Read the model definition and answer for the solid it produces. Units are mm, in the model's axes. A direction names the side the tool comes from. Coordinates: 2 decimals unless noted, no trailing zeros. Loops run counter-clockwise (first coordinate to the right, second up) from the corner with the lowest first, then second, coordinate; pieces in that order, holes last.
from build123d import *

# Parameters (mm, degrees)
SKETCH1_R           = 1.3
BOSS_EXTRUDE1_DEPTH = 2.8
BOSS_EXTRUDE2_START = -1.8
SKETCH2_R           = 1.3
BOSS_EXTRUDE2_DEPTH = 1.8
SKETCH3_R           = 2.25
CUT_EXTRUDE1_DEPTH  = 2.5
SKETCH4_W           = 35.6
SKETCH4_H           = 4.6
BOSS_EXTRUDE3_DEPTH = 5
SKETCH5_W           = 4.5
SKETCH5_H           = 35.6
BOSS_EXTRUDE4_DEPTH = 15
FILLET1_R           = 1
CUT_EXTRUDE4_DEPTH  = 3.5
SKETCH10_R          = 30
BOSS_EXTRUDE6_DEPTH = 4.5
SKETCH6_R           = 1.6
CUT_EXTRUDE2_DEPTH  = 69.491291157
SKETCH8_R           = 2.8
CUT_EXTRUDE3_DEPTH  = 2.7
RIB1_REACH          = 73.132
SKETCH11_WALL_W     = 161.35156572
SKETCH11_WALL_H     = 8
FILLET2_R           = 0.5
FILLET3_R           = 0.5


with BuildPart() as part:
    # Sketch1 → Boss-Extrude1 (new body)
    with BuildSketch(Plane(origin=(0, 0, 0), x_dir=(1, 0, 0), z_dir=(0, 1, 0))):
        Polygon((4.489988864, 12.2), (4.489988864, 17.8), (38.3, 17.8), (38.3, -17.8), (4.489988864, -17.8), (4.489988864, -12.2), (33.2, -12.2), (33.2, 12.2), align=None)
        with Locations(Location((12.5, 15, 0), (0, 0, 270))):
            Circle(SKETCH1_R, mode=Mode.SUBTRACT)
        with Locations(Location((29.5, 15, 0), (0, 0, 270))):
            Circle(SKETCH1_R, mode=Mode.SUBTRACT)
        with Locations(Location((12.5, -15, 0), (0, 0, 270))):
            Circle(SKETCH1_R, mode=Mode.SUBTRACT)
        with Locations(Location((29.5, -15, 0), (0, 0, 270))):
            Circle(SKETCH1_R, mode=Mode.SUBTRACT)
        with Locations(Location((35.75, -8.5, 0), (0, 0, 270))):
            Circle(SKETCH1_R, mode=Mode.SUBTRACT)
        with Locations(Location((35.75, 8.5, 0), (0, 0, 270))):
            Circle(SKETCH1_R, mode=Mode.SUBTRACT)
    boss_extrude1 = extrude(amount=BOSS_EXTRUDE1_DEPTH)

    # Sketch2 → Boss-Extrude2 (add)
    # profile 1 of 2: a face of its own
    with BuildSketch(Plane(origin=(0, 0, 0), x_dir=(1, 0, 0), z_dir=(0, 1, 0)).offset(BOSS_EXTRUDE2_START)):
        with BuildLine():
            ThreePointArc((4.489988864, -12.2), (13, 0), (4.489988864, 12.2))
            Line((4.489988864, 12.2), (33.2, 12.2))
            Line((33.2, 12.2), (33.2, -12.2))
            Line((33.2, -12.2), (4.489988864, -12.2))
        make_face()
    # profile 2 of 2: a face of its own
    with BuildSketch(Plane(origin=(0, 0, 0), x_dir=(1, 0, 0), z_dir=(0, 1, 0)).offset(BOSS_EXTRUDE2_START)):
        Polygon((4.489988864, 12.2), (4.489988864, 17.8), (38.3, 17.8), (38.3, -17.8), (4.489988864, -17.8), (4.489988864, -12.2), (33.2, -12.2), (33.2, 12.2), align=None)
        with Locations(Location((12.5, -15, 0), (0, 0, 270))):
            Circle(SKETCH2_R, mode=Mode.SUBTRACT)
        with Locations(Location((29.5, -15, 0), (0, 0, 270))):
            Circle(SKETCH2_R, mode=Mode.SUBTRACT)
        with Locations(Location((35.75, -8.5, 0), (0, 0, 270))):
            Circle(SKETCH2_R, mode=Mode.SUBTRACT)
        with Locations(Location((35.75, 8.5, 0), (0, 0, 270))):
            Circle(SKETCH2_R, mode=Mode.SUBTRACT)
        with Locations(Location((29.5, 15, 0), (0, 0, 270))):
            Circle(SKETCH2_R, mode=Mode.SUBTRACT)
        with Locations(Location((12.5, 15, 0), (0, 0, 270))):
            Circle(SKETCH2_R, mode=Mode.SUBTRACT)
    boss_extrude2 = extrude(amount=BOSS_EXTRUDE2_DEPTH)

    # Sketch3 → Cut-Extrude1 (cut)
    with BuildSketch(Plane.XZ.offset(1.8)):
        with Locations(Location((12.5, 15, 0), (0, 0, 270))):
            Circle(SKETCH3_R)
        with Locations(Location((29.5, 15, 0), (0, 0, 270))):
            Circle(SKETCH3_R)
        with Locations(Location((29.5, -15, 0), (0, 0, 270))):
            Circle(SKETCH3_R)
        with Locations(Location((12.5, -15, 0), (0, 0, 270))):
            Circle(SKETCH3_R)
        with Locations(Location((35.75, 8.5, 0), (0, 0, 270))):
            Circle(SKETCH3_R)
        with Locations(Location((35.75, -8.5, 0), (0, 0, 270))):
            Circle(SKETCH3_R)
    cut_extrude1 = extrude(amount=-CUT_EXTRUDE1_DEPTH, mode=Mode.SUBTRACT)

    # Sketch4 → Boss-Extrude3 (add)
    with BuildSketch(Plane(origin=(38.3, 0, 0), x_dir=(0, 0, -1), z_dir=(1, 0, 0))):
        with Locations((0, 0.5)):
            Rectangle(SKETCH4_W, SKETCH4_H)
    boss_extrude3 = extrude(amount=BOSS_EXTRUDE3_DEPTH)

    # Sketch5 → Boss-Extrude4 (add)
    with BuildSketch(Plane(origin=(0, 2.8, 0), x_dir=(1, 0, 0), z_dir=(0, 1, 0))):
        with Locations((41.05, 0)):
            Rectangle(SKETCH5_W, SKETCH5_H)
    boss_extrude4 = extrude(amount=BOSS_EXTRUDE4_DEPTH)

    # Mirror3: Boss-Extrude1, Boss-Extrude2, Cut-Extrude1, Boss-Extrude3, Boss-Extrude4 across plane
    add(boss_extrude1.mirror(Plane.ZX.offset(17.8)))
    add(boss_extrude2.mirror(Plane.ZX.offset(17.8)))
    add(cut_extrude1.mirror(Plane.ZX.offset(17.8)), mode=Mode.SUBTRACT)
    add(boss_extrude3.mirror(Plane.ZX.offset(17.8)))
    add(boss_extrude4.mirror(Plane.ZX.offset(17.8)))

    # Fillet1
    fillet1_edges = [part.edges().sort_by_distance(p)[0] for p in [
        (4.489988864, 35.1, -17.8),
        (4.489988864, 35.1, 17.8),
        (4.489988864, 0.5, 17.8),
        (4.489988864, 0.5, -17.8),
    ]]
    fillet(fillet1_edges, radius=FILLET1_R)

    # Sketch9 → Cut-Extrude4 (cut)
    with BuildSketch(Plane(origin=(43.3, 0, 0), x_dir=(0, 0, -1), z_dir=(1, 0, 0))):
        with BuildLine():
            Line((-2.05, 21.85), (2.05, 21.85))
            ThreePointArc((2.05, 21.85), (3.464213562, 21.264213562), (4.05, 19.85))
            Line((4.05, 19.85), (4.05, 15.75))
            ThreePointArc((4.05, 15.75), (3.464213562, 14.335786438), (2.05, 13.75))
            Line((2.05, 13.75), (-2.05, 13.75))
            ThreePointArc((-2.05, 13.75), (-3.464213562, 14.335786438), (-4.05, 15.75))
            Line((-4.05, 15.75), (-4.05, 19.85))
            ThreePointArc((-4.05, 19.85), (-3.464213562, 21.264213562), (-2.05, 21.85))
        make_face()
    extrude(amount=-CUT_EXTRUDE4_DEPTH, mode=Mode.SUBTRACT)

    # Sketch10 → Boss-Extrude6 (add)
    with BuildSketch(Plane.ZY.offset(-38.8)):
        with Locations((0, 17.8)):
            Circle(SKETCH10_R)
    extrude(amount=-BOSS_EXTRUDE6_DEPTH)

    # Sketch6 → Cut-Extrude2 (cut, through all)
    with BuildSketch(Plane(origin=(43.3, 0, 0), x_dir=(0, 0, -1), z_dir=(1, 0, 0))):
        with Locations((-8.485281374, 26.285281374)):
            Circle(SKETCH6_R)
        with Locations((8.485281374, 26.285281374)):
            Circle(SKETCH6_R)
        with Locations((8.485281374, 9.314718626)):
            Circle(SKETCH6_R)
        with Locations((-8.485281374, 9.314718626)):
            Circle(SKETCH6_R)
    extrude(amount=-CUT_EXTRUDE2_DEPTH, mode=Mode.SUBTRACT)

    # Sketch8 → Cut-Extrude3 (cut)
    with BuildSketch(Plane.ZY.offset(-38.8)):
        with Locations((-8.485281374, 26.285281374)):
            Circle(SKETCH8_R)
        with Locations((8.485281374, 26.285281374)):
            Circle(SKETCH8_R)
        with Locations((8.485281374, 9.314718626)):
            Circle(SKETCH8_R)
        with Locations((-8.485281374, 9.314718626)):
            Circle(SKETCH8_R)
    extrude(amount=-CUT_EXTRUDE3_DEPTH, mode=Mode.SUBTRACT)

    # Sketch11 wall → Rib1 (add, up to next)
    with BuildSketch(Plane(origin=(30.8, 40.4, 0), x_dir=(-0.936329177569, -0.351123441588, 0), z_dir=(0.351123441588, -0.936329177569, 0)), mode=Mode.PRIVATE) as rib1_sk1:
        Rectangle(SKETCH11_WALL_W, SKETCH11_WALL_H)
    rib1_tool1 = extrude(rib1_sk1.sketch, amount=RIB1_REACH, mode=Mode.PRIVATE) - part.part
    rib1 = rib1_tool1.solids().sort_by_distance((30.8, 40.4, 0))[0]
    add(rib1)

    # Mirror4: Rib1 across plane
    add(rib1.mirror(Plane.ZX.offset(17.8)))

    # Fillet2
    fillet2_edges = [part.edges().sort_by_distance(p)[0] for p in [
        (38.8, 17.8, -30),
    ]]
    fillet(fillet2_edges, radius=FILLET2_R)

    # Fillet3
    fillet3_edges = [part.edges().sort_by_distance(p)[0] for p in [
        (4.489988864, 37.4, -14.5),
        (22.144994432, -1.8, -17.8),
        (22.144994432, -1.8, 17.8),
        (4.489988864, -1.8, 14.5),
        (4.782882083, -1.8, 17.507106781),
        (4.782882083, -1.8, -17.507106781),
        (22.144994432, 37.4, -17.8),
        (4.489988864, 37.4, 14.5),
        (22.144994432, 37.4, 17.8),
        (4.782882083, 37.4, 17.507106781),
        (4.782882083, 37.4, -17.507106781),
        (38.8, 37.4, 10.9),
        (38.8, -1.8, -10.9),
        (38.8, 0.5, 17.8),
        (38.8, 35.1, 17.8),
        (38.8, 0.5, -17.8),
        (38.8, 35.1, -17.8),
        (38.8, 37.4, -10.9),
        (38.8, 43.4, 0),
        (38.8, 40.4, 4),
        (38.8, 40.4, -4),
        (38.8, -1.8, 10.9),
        (38.8, -7.8, 0),
        (38.8, -4.8, 4),
        (38.8, -4.8, -4),
        (4.489988864, -1.8, -14.5),
    ]]
    fillet(fillet3_edges, radius=FILLET3_R)


solid = part.part
Item 1: Given pin 1 (10 mm diameter, centred on x = 30.5, z = -16, fed in from +Y); pin 2 (5 mm diameter, centred on x = 29.5, z = 15, fed in from -Y); pin 3 (4 mm diameter, centred on x = 9, y = 2.5, fed in from +Z); pin 4 (3 mm diameter, centred on y = 9.31, z = 8.49, fed in from +X), each flat-ended and moving along its own axis, determine where each tip first touches the part or whether it passes through.
Numbers:
pin 1: stops at y = 37.4
pin 2: stops at y = -1.8
pin 3: stops at z = 17.8
pin 4: passes through
Item 2: Find the intervals of material crossed by line 1 along X through (y, z) = (1.2, -8.5); line 2 along X through (y, z) = (35.85, 15); line 3 along Z through (x, y) = (35, 33), in increasing order.
Numbers:
line 1: x = 33.2 to 34.45, 37.05 to 43.3
line 2: x = 4.49 to 10.25, 14.75 to 27.25, 31.75 to 43.3
line 3: z = -17.8 to -9.56, -7.44 to 7.44, 9.56 to 17.8
Item 3: A cutting plane is placed at A-A on x = 20. Determine the outline of the cut face in (y, z), then the cut area to 3 significant figures.
Numbers:
outline: (-1.8, -17.3) arc R0.5 ccw to (-1.3, -17.8) - (2.8, -17.8) - (2.8, -12.2) - (0, -12.2) - (0, 12.2) - (2.8, 12.2) - (2.8, 17.8) - (-1.3, 17.8) arc R0.5 ccw to (-1.8, 17.3) - close; (32.8, -17.8) - (36.9, -17.8) arc R0.5 ccw to (37.4, -17.3) - (37.4, 17.3) arc R0.5 ccw to (36.9, 17.8) - (32.8, 17.8) - (32.8, 12.2) - (35.6, 12.2) - (35.6, -12.2) - (32.8, -12.2) - close
area: 191 mm2
Item 4: A cutting plane is placed at B-B on z = 0. Determine the outline of the cut face in (x, y).
Numbers:
outline: (13, -1.8) - (22.8, -1.8) - (38.48, -7.68) arc R0.5 cw to (38.8, -8.15) - (38.8, -11.7) arc R0.5 ccw to (39.3, -12.2) - (43.3, -12.2) - (43.3, 47.8) - (39.3, 47.8) arc R0.5 ccw to (38.8, 47.3) - (38.8, 43.75) arc R0.5 cw to (38.48, 43.28) - (22.8, 37.4) - (13, 37.4) - (13, 35.6) - (33.2, 35.6) - (33.2, 32.8) - (38.8, 32.8) - (38.8, 2.8) - (33.2, 2.8) - (33.2, 0) - (13, 0) - close
Item 5: Which of the six approach directions +Z, -Z, +X, -X, +Y, -Y give full straight-line access (tool end or side, diameter ignored) to faces 1 (the face through (22, 0, 0)), 2 (the face through (14.397, 36.168, 13.79)), 3 (the face through (29.5, 0.7, 13.5)), 4 (the face through (22, 1, -17.8))?
Numbers:
face 1: -X
face 2: +Y
face 3: -Y
face 4: -Z, -X, +Y, -Y
Item 6: Determine the mould class of faces 5 (the face through (33, 40, -4)), 6 (the face through (37.98, 36.17, -8.21)), 7 (the face through (4.49, 35, -14)) for opening direction Z: released by +Z, released by -Z, zero draft, split by the parting line, or undercut.
Numbers:
face 5: released by -Z
face 6: undercut
face 7: zero draft
Item 7: A cutting plane is placed at C-C on z = 15.5. Give the number of separate pieces and of enclosed holes in the cut face, then the cut area to 3 significant figures.
Numbers:
separate pieces: 5
enclosed holes: 0
area: 483 mm2
